from build123d import *

# Parameters (mm, degrees)
F0_W         = 12.7
F0_H         = 12.7
F1_DEPTH     = 38.1
F2_R         = 5.08
F3_W         = 25.4
F3_H         = 25.4
F4_DEPTH     = 12.7
F6_DEPTH     = 6.35
F8_R         = 5.08
F9_T1_DEPTH  = 45.72
F9_T3_DEPTH  = 50.8
F10_T1_DEPTH = 45.72
F10_T3_DEPTH = 50.8


# Not quite as in the source:
# - a fillet or chamfer that OpenCascade refuses, or shapes differently, is made with other operations: its cross-section is extruded or revolved along the edge and cut away or added


with BuildPart() as f1:
    # F0 (on Right) → F1 (new body)
    with BuildSketch(Plane.YZ):
        Rectangle(F0_W, F0_H)
    extrude(amount=F1_DEPTH)

    # F2
    f2_edges = [f1.edges().sort_by_distance(p)[0] for p in [
        (19.05, 6.35, 6.35),
        (19.05, -6.35, 6.35),
        (0, 0, 6.35),
    ]]
    fillet(f2_edges, radius=F2_R)

    # F3 (on Right) → F4 (join)
    with BuildSketch(Plane.YZ):
        with Locations((0, 1.27)):
            Rectangle(F3_W, F3_H)
    extrude(amount=F4_DEPTH)

    # F5 (on face) → F6 (join)
    with BuildSketch(Plane.YZ.offset(38.1)):
        Polygon((-18.3308710468, -31.75), (18.3308710468, -31.75), (36.6617420935, 0), (18.3308710468, 31.75), (-18.3308710468, 31.75), (-36.6617420935, 0), align=None)
    extrude(amount=-F6_DEPTH)

    # F7: F1 across plane


with BuildPart() as f1_1:
    add(f1.part)
    add(f1.part.mirror(Plane.YZ))

    # F8
    f8_edges = [f1_1.edges().sort_by_distance(p)[0] for p in [
        (12.7, 0, 13.97),
        (0, -12.7, 13.97),
        (-12.7, 0, 13.97),
        (0, 12.7, 13.97),
    ]]
    fillet(f8_edges, radius=F8_R)

    # F9: fillet of radius 5.08 on 4 edges, made by hand

    # F9_s2 → F9_t1 (cut)
    with BuildSketch(Plane.XY.offset(-24.13)):
        with BuildLine():
            ThreePointArc((12.7, -7.62), (11.2121024484, -11.2121024484), (7.62, -12.7))
            Line((7.62, -12.7), (12.7, -12.7))
            Line((12.7, -12.7), (12.7, -7.62))
        make_face()
        with BuildLine():
            ThreePointArc((-7.62, -12.7), (-11.2121024484, -11.2121024484), (-12.7, -7.62))
            Line((-12.7, -7.62), (-12.7, -12.7))
            Line((-12.7, -12.7), (-7.62, -12.7))
        make_face()
    extrude(amount=F9_T1_DEPTH, mode=Mode.SUBTRACT)

    # F9_s4 → F9_t3 (cut)
    with BuildSketch(Plane.YZ.offset(-25.4)):
        with BuildLine():
            ThreePointArc((-7.62, -11.43), (-11.2121024484, -9.9421024484), (-12.7, -6.35))
            Line((-12.7, -6.35), (-12.7, -11.43))
            Line((-12.7, -11.43), (-7.62, -11.43))
        make_face()
    extrude(amount=F9_T3_DEPTH, mode=Mode.SUBTRACT)

    # F10: fillet of radius 5.08 on 4 edges, made by hand

    # F10_s2 → F10_t1 (cut)
    with BuildSketch(Plane.XY.offset(-24.13)):
        with BuildLine():
            ThreePointArc((12.7, 7.62), (11.2121024484, 11.2121024484), (7.62, 12.7))
            Line((7.62, 12.7), (12.7, 12.7))
            Line((12.7, 12.7), (12.7, 7.62))
        make_face()
        with BuildLine():
            ThreePointArc((-7.62, 12.7), (-11.2121024484, 11.2121024484), (-12.7, 7.62))
            Line((-12.7, 7.62), (-12.7, 12.7))
            Line((-12.7, 12.7), (-7.62, 12.7))
        make_face()
    extrude(amount=F10_T1_DEPTH, mode=Mode.SUBTRACT)

    # F10_s4 → F10_t3 (cut)
    with BuildSketch(Plane.YZ.offset(-25.4)):
        with BuildLine():
            ThreePointArc((12.7, -6.35), (11.2121024484, -9.9421024484), (7.62, -11.43))
            Line((7.62, -11.43), (12.7, -11.43))
            Line((12.7, -11.43), (12.7, -6.35))
        make_face()
    extrude(amount=F10_T3_DEPTH, mode=Mode.SUBTRACT)


solid = f1_1.part
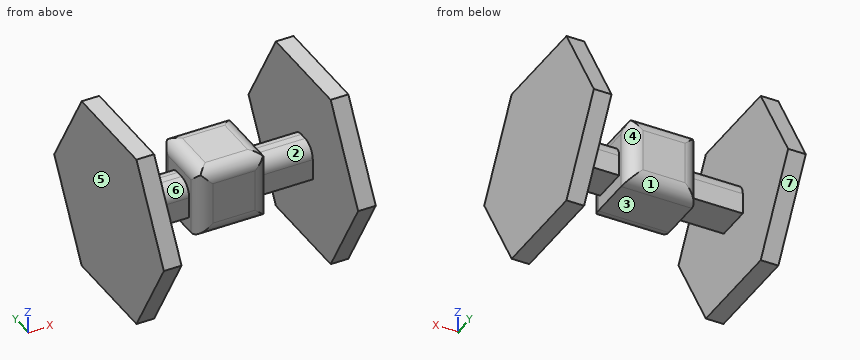
Input: part model. Units: mm. Frame: model coordinates. Face numbers are marked on the shaded views. A direction names the side the tool comes from. Round coordinates to 2 decimals unless told otherwise and drop trailing zeros. Write each loop counter-clockwise with the first axis right and the second up, starting at its lowest first coordinate (ties: lowest second). Pieces come first, ordered by that corner, then holes.
1) Cut plane A-A (y = 16). Return the cut outline in (x, z), then the cut area to 3 significant figures.
2) Cut plane B-B (z = -13). Return the cut outline in (x, y), then the cut area to 3 significant figures.
3) Reachability of the marked faces 1, 2, 3 and 4 from +Z, -Z, +X, -X, +Y, -Y: full face, straight path, thin tool, end or side. Return the list, or none.
4) Contact query for flat-ended pins moving along their axis: P1, Ø17, axis at x = -2.5, z = 1, coming from the +Y side; P2, Ø8, axis at x = -9.5, y = -7.5, coming from the -Z side; P3, Ø6.5, axis at x = -18, y = 0.5, coming from the -Z side. Output: stop coordinate, or through.
5) Cut plane C-C (x = 18.5). Return the cut outline in (y, z), then the cut area to 3 significant figures.
6) Draft query along X for the marked faces 5, 6 and 7. Return one class per face: pulls with the +X half, pulls with the -X half, needs draft (parallel to the pull), parting line crosses it, or undercut.
7) Ray query, L1, parallel to X at y = -13, z = 25; L2, parallel to Z at x = -0.5, y = -5.5; L3, parallel to Y at x = 7.5, z = -8. Return the intervals inside material, ascending.
8) Cut plane D-D (y = 0). Return the cut outline in (x, z), then the cut area to 3 significant figures.
Geometry says:
1. outline: (-38.1, -31.75) - (-31.75, -31.75) - (-31.75, 31.75) - (-38.1, 31.75) - close; (31.75, -31.75) - (38.1, -31.75) - (38.1, 31.75) - (31.75, 31.75) - close
1. area: 806 mm2
2. outline: (-38.1, -29.16) - (-31.75, -29.16) - (-31.75, 29.16) - (-38.1, 29.16) - close; (31.75, -29.16) - (38.1, -29.16) - (38.1, 29.16) - (31.75, 29.16) - close
2. area: 741 mm2
3. face 1: -Z, +Y
3. face 2: +Z, -Y
3. face 3: -Z, +Y, -Y
3. face 4: +Z, -Z, +Y
4. P1: stops at y = 12.7
4. P2: stops at z = -11.43
4. P3: stops at z = -6.35
5. outline: (-6.35, -6.35) - (6.35, -6.35) - (6.35, 1.27) arc R5.08 ccw to (1.27, 6.35) - (-1.27, 6.35) arc R5.08 ccw to (-6.35, 1.27) - close
5. area: 150 mm2
6. face 5: pulls with the -X half
6. face 6: undercut
6. face 7: needs draft
7. L1: x = -38.1 to -31.75, 31.75 to 38.1
7. L2: z = -11.43 to 13.97
7. L3: y = -12.42 to 12.42
8. outline: (-38.1, -31.75) - (-31.75, -31.75) - (-31.75, -6.35) - (-12.7, -6.35) - (-12.7, -11.43) - (12.7, -11.43) - (12.7, -6.35) - (31.75, -6.35) - (31.75, -31.75) - (38.1, -31.75) - (38.1, 31.75) - (31.75, 31.75) - (31.75, 6.35) - (12.7, 6.35) - (12.7, 8.89) arc R5.08 ccw to (7.62, 13.97) - (-7.62, 13.97) arc R5.08 ccw to (-12.7, 8.89) - (-12.7, 6.35) - (-31.75, 6.35) - (-31.75, 31.75) - (-38.1, 31.75) - close
8. area: 1,920 mm2
